Read the model definition and answer for the solid it produces. Units are mm, in the model's axes. Face numbers are marked on the shaded views. A direction names the side the tool comes from. Coordinates: 2 decimals unless noted, no trailing zeros. Order: outer loops, then holes, each group sorted by start corner. A loop starts at its lowest first (then second) coordinate and runs counter-clockwise, first axis right, second up. Notation, with made-up numbers: (12.25, -33.5) -> (30.25, -33.5) arc R3 cw to (30.25, -28.5) -> close; hole circle Ø6 at (1, -22.5). An arc over 180 degrees is marked (long way). Return JSON: item names as keys, results as strings. Group by question number.
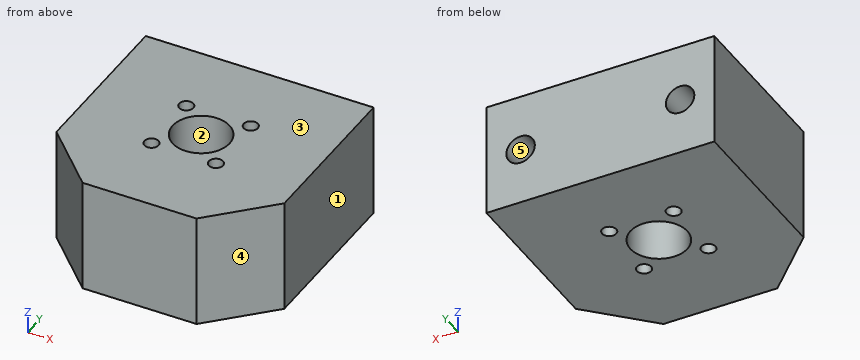
```python
from build123d import *

# Parameters (mm, degrees)
F0_W     = 40
F0_H     = 39
F0_R     = 1.25
F0_R_2   = 5
F1_DEPTH = 20
F2_SIZE  = 10
F3_R     = 2.5
F4_DEPTH = 25


with BuildPart() as f1:
    # F0 (on Top) → F1 (new body)
    with BuildSketch(Plane.XY):
        Rectangle(F0_W, F0_H)
        with Locations((-5.656854, -5.156854)):
            Circle(F0_R, mode=Mode.SUBTRACT)
        with Locations((5.656854, -5.156854)):
            Circle(F0_R, mode=Mode.SUBTRACT)
        with Locations((-5.656854, 6.156854)):
            Circle(F0_R, mode=Mode.SUBTRACT)
        with Locations((0, 0.5)):
            Circle(F0_R_2, mode=Mode.SUBTRACT)
        with Locations((5.656854, 6.156854)):
            Circle(F0_R, mode=Mode.SUBTRACT)
    extrude(amount=F1_DEPTH)

    # F2
    f2_edges = [f1.edges().sort_by_distance(p)[0] for p in [
        (-20, -19.5, 10),
        (20, -19.5, 10),
    ]]
    chamfer(f2_edges, length=F2_SIZE)

    # F3 (on face) → F4 (cut)
    with BuildSketch(Plane(origin=(0, 19.5, 0), x_dir=(-1, 0, 0), z_dir=(0, 1, 0))):
        with Locations((14, 10)):
            Circle(F3_R)
        with Locations((-14, 10)):
            Circle(F3_R)
    extrude(amount=-F4_DEPTH, mode=Mode.SUBTRACT)


solid = f1.part
```
1. Given pin 1 (3 mm diameter, centred on x = -5.66, y = 6.16, fed in from +Z); pin 2 (4 mm diameter, centred on x = 14, z = 10, fed in from +Y); pin 3 (4.5 mm diameter, centred on x = -14, z = 10, fed in from -Y), each flat-ended and moving along its own axis, determine where each tip first touches the part or whether it passes through.
2. Find section B-B on x = 16. Determine the outline of the cut face in (y, z).
3. Find section D-D on z = 13.5. Determine the outline of the cut face in (x, y).
4. For a pull along X with two mould halves and no side action, classify the marked faces 1, 2 and 3 as released by +X, released by -X, zero draft, split by the parting line, or undercut.
5. Find section C-C on y = 10. Determine the outline of the cut face in (x, z).
6. Find section A-A on y = 0.5. Determine the outline of the cut face in (x, z), and give its area (3 significant figures).
7. Straight lines are drawn through the part: L1, parallel to X at y = 16.5, z = 9.75; L2, parallel to Y at x = -5.5, z = 18.5; L3, parallel to X at y = 11, z = 10.75. For each, find the intervals that lie inside material, in ascending order.
8. Which of the six approach directions +Z, -Z, +X, -X, +Y, -Y give full straight-line access (tool end or side, diameter ignored) to the marked faces 4 and 5?
Result:
{
 "1": {"pin 1": "z = 20", "pin 2": "y = -5.5", "pin 3": "y = -17.75"},
 "2": {"outline": "(-13.5, 0) -> (19.5, 0) -> (19.5, 8.5) -> (-5.5, 8.5) -> (-5.5, 11.5) -> (19.5, 11.5) -> (19.5, 20) -> (-13.5, 20) -> close"},
 "3": {"outline": "(-20, -9.5) -> (-10, -19.5) -> (10, -19.5) -> (20, -9.5) -> (20, 19.5) -> (-20, 19.5) -> close; hole circle Ø2.5 at (-5.66, -5.16); hole circle Ø2.5 at (-5.66, 6.16); hole circle Ø10 at (0, 0.5); hole circle Ø2.5 at (5.66, -5.16); hole circle Ø2.5 at (5.66, 6.16)"},
 "4": {"face 1": "released by +X", "face 2": "undercut", "face 3": "zero draft"},
 "5": {"outline": "(-20, 0) -> (20, 0) -> (20, 20) -> (-20, 20) -> close; hole circle Ø5 at (-14, 10); hole circle Ø5 at (14, 10)"},
 "6": {"outline": "(-20, 0) -> (-5, 0) -> (-5, 20) -> (-20, 20) -> close; (5, 0) -> (20, 0) -> (20, 20) -> (5, 20) -> close; hole circle Ø5 at (-14, 10); hole circle Ø5 at (14, 10)", "area": "561 mm^2"},
 "7": {"L1": "-20 to -16.49, -11.51 to 11.51, 16.49 to 20", "L2": "-19.5 to -6.4, -3.92 to 4.92, 7.4 to 19.5", "L3": "-20 to -16.38, -11.62 to 11.62, 16.38 to 20"},
 "8": {"face 4": "+Z, -Z, +X, -Y", "face 5": "+Y"}
}
